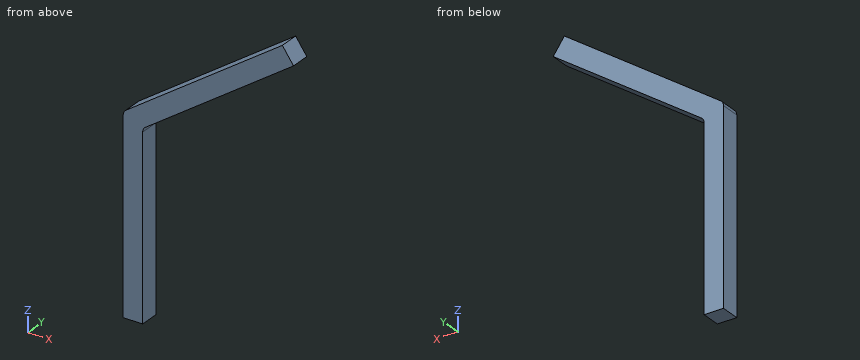
from build123d import *

# Parameters (mm, degrees)
F1_DEPTH = 3
F2_R     = 1


with BuildPart() as f1:
    # F0 (on Front) → F1 (new body)
    with BuildSketch(Plane.XZ):
        Polygon((0, 30), (0, 0), (3, 0), (3, 28.438299), (1.720729, 27.542544), align=None)
        Polygon((3, 30), (0, 30), (1.720729, 27.542544), (3, 28.438299), align=None)
        Polygon((24.574561, 47.207293), (0, 30), (3, 30), (3, 28.438299), (26.295291, 44.749837), align=None)
    extrude(amount=F1_DEPTH)

    # F2
    f2_edges = [f1.edges().sort_by_distance(p)[0] for p in [
        (0, -1.5, 30),
        (3, -1.5, 28.438299),
    ]]
    fillet(f2_edges, radius=F2_R)


solid = f1.part
Model file for the job. Use its own axes, mm. Give positions to 0.01 mm unless a question says otherwise; leave off trailing zeros. Write each loop counter-clockwise with the first axis right and the second up, starting at its lowest first coordinate (ties: lowest second). Pieces come first, ordered by that corner, then holes. Notation, with made-up numbers: (62, -17) - (103, -17) arc R22 cw to (103, 1) - close; hole circle Ø6 at (-15, 76). An arc over 180 degrees is marked (long way). Answer as CSV lines item,"result".
1. Drill centre lines: L1, parallel to X at y = -0.7, z = 3; L2, parallel to X at y = -1.05, z = 42.5; L3, parallel to Z at x = 12, y = -2.3. Where is each one in solid material? Low to high. Write a range as [from, to].
Responses:
L1,"x = [0, 3]"
L2,"x = [17.85, 23.08]"
L3,"z = [34.74, 38.4]"
2. Pin check, flat tips, straight feed: pin 1 (1.5 mm diameter, centred on y = -1, z = 13, fed in from +X); pin 2 (1.5 mm diameter, centred on x = 21, y = -2.5, fed in from -Z); pin 3 (8 mm diameter, centred on x = 7.5, z = 20.5, fed in from +Y). Stop position of each tip, or through.
Responses:
pin 1,"stops at x = 3"
pin 2,"stops at z = 40.52"
pin 3,"passes through"
3. Band-saw the part on A-A (y = -0.6). Write the cut outline in (x, z), and give its area (3 significant figures).
Responses:
outline,"(0, 0) - (3, 0) - (3, 27.92) arc R1 cw to (3.43, 28.74) - (26.3, 44.75) - (24.57, 47.21) - (0.43, 30.3) arc R1 ccw to (0, 29.48) - close"
area,"175 mm2"
4. Band-saw the part on B-B (z = 15.5). Write the cut outline in (x, y).
Responses:
outline,"(0, -3) - (3, -3) - (3, 0) - (0, 0) - close"
5. Band-saw the part on C-C (x = 8.25). Write the cut outline in (y, z), and give its area (3 significant figures).
Responses:
outline,"(-3, 32.11) - (0, 32.11) - (0, 35.78) - (-3, 35.78) - close"
area,"11.0 mm2"
